Work out the finished part from the listing and answer in its coordinate system (mm). A direction names the side the tool comes from. Round coordinates to 2 decimals unless told otherwise and drop trailing zeros. Loops run counter-clockwise (first coordinate to the right, second up) from the corner with the lowest first, then second, coordinate; pieces in that order, holes last.
from build123d import *

# Parameters (mm, degrees)
BOSS_EXTRUDE1_DEPTH = 2.032
BOSS_EXTRUDE2_DEPTH = 5.7
CUT_EXTRUDE1_DEPTH  = 7
FILLET1_R           = 0.6


with BuildPart() as part:
    # Sketch1 → Boss-Extrude1 (new body)
    with BuildSketch(Plane.XY):
        with BuildLine():
            Line((3.81, 0), (3.81, -180.234))
            Line((3.81, -180.234), (2.654016147, -213.337046398))
            ThreePointArc((2.654016147, -213.337046398), (1.844758309, -215.154669263), (0, -215.9))
            Line((0, -215.9), (0, 0))
            Line((0, 0), (3.81, 0))
        make_face()
    extrude(amount=BOSS_EXTRUDE1_DEPTH)

    # Sketch5 → Boss-Extrude2 (add)
    with BuildSketch(Plane.ZY):
        Polygon((0, 0), (7, 0), (7, -9.187579355), (0, -9.8), align=None)
    extrude(amount=-BOSS_EXTRUDE2_DEPTH)

    # Sketch4 → Cut-Extrude1 (cut)
    with BuildSketch(Plane.XY.offset(7)):
        Polygon((0, -3.8), (3.8, -3.8), (3.8, -6), (2.85, -6), (2.85, -5.05), (0, -5.05), align=None)
    extrude(amount=-CUT_EXTRUDE1_DEPTH, mode=Mode.SUBTRACT)

    # Fillet1
    fillet1_edges = [part.edges().sort_by_distance(p)[0] for p in [
        (5.7, 0, 3.5),
        (5.7, -9.493789678, 3.5),
    ]]
    fillet(fillet1_edges, radius=FILLET1_R)

    # Mirror1: part across plane


with BuildPart() as part_1:
    add(part.part)
    add(part.part.mirror(Plane(origin=(0, -215.9, 2.032), x_dir=(0, 0, 1), z_dir=(1, 0, 0))))


solid = part_1.part
Item 1: For faces 1 (the face through (0, -3.8, 4)), 2 (the face through (0, -106, 0)), 3 (the face through (0, -111, 2.032)), determine the directions among +Z, -Z, +X, -X, +Y, -Y from which every point of the face is accessible in a straight line to the end or side of a thin tool.
Item 2: Each of these flat-tipped pins is pushed along its axis until it touches: P1, Ø3, axis at y = -99.5, z = 4.5, coming from the +X side; P2, Ø0.6, axis at y = -116, z = 0.5, coming from the -X side; P3, Ø1, axis at x = 3.5, y = -83, coming from the +Z side; P4, Ø1, axis at y = -84, z = 1, coming from the +X side. Where does it stop, or does it pass through?
Item 3: Determine the mould class of faces 4 (the face through (0, -5.05, 4)), 5 (the face through (0, 0, 3)), 6 (the face through (0.1, -3.5, 7)) for opening direction Y: pulls with the +Y half, pulls with the -Y half, needs draft (parallel to the pull), parting line crosses it, or undercut.
Item 4: Section B-B, the plane y = -202 is taken. Give the vertices of the cut face in (x, z), plus the area to 3 significant figures.
Item 5: Straight lines are drawn through the part: line 1 (Y direction, x = 2, z = 2.5); line 2 (Y direction, x = 2.75, z = 6.5); line 3 (X direction, y = -54.5, z = 1). For each, find the intervals that lie inside material, in ascending order.
Item 6: Section A-A, the plane y = -175 is taken. Give the vertices of the cut face in (x, z), plus the area to 3 significant figures.
Answer below:
1. face 1: +Z, -Z
1. face 2: -Z, +X, -X, +Y, -Y
1. face 3: +Z, +X, -X, -Y
2. P1: passes through
2. P2: stops at x = -3.81
2. P3: stops at z = 2.03
2. P4: stops at x = 3.81
3. face 4: undercut
3. face 5: pulls with the +Y half
3. face 6: needs draft
4. outline: (-3.05, 0) - (3.05, 0) - (3.05, 2.03) - (-3.05, 2.03) - close
4. area: 12.4 mm2
5. line 1: y = -9.58 to -5.05, -3.8 to 0
5. line 2: y = -9.23 to -5.05, -3.8 to 0
5. line 3: x = -3.81 to 3.81
6. outline: (-3.81, 0) - (3.81, 0) - (3.81, 2.03) - (-3.81, 2.03) - close
6. area: 15.5 mm2
